Verification items for this drawing (mm, ordinates from the low corner). A direction names the side the tool comes from. Round coordinates to 2 decimals unless told otherwise and drop trailing zeros. Loops run counter-clockwise (first coordinate to the right, second up) from the corner with the lowest first, then second, coordinate; pieces in that order, holes last. Notation, with made-up numbers: (26, 3) - (63, 3) arc R21 cw to (63, 37) - close; hole circle Ø8 at (33, 73). An arc over 180 degrees is marked (long way). Put each result on its own line as item: value. Start each with the question number.
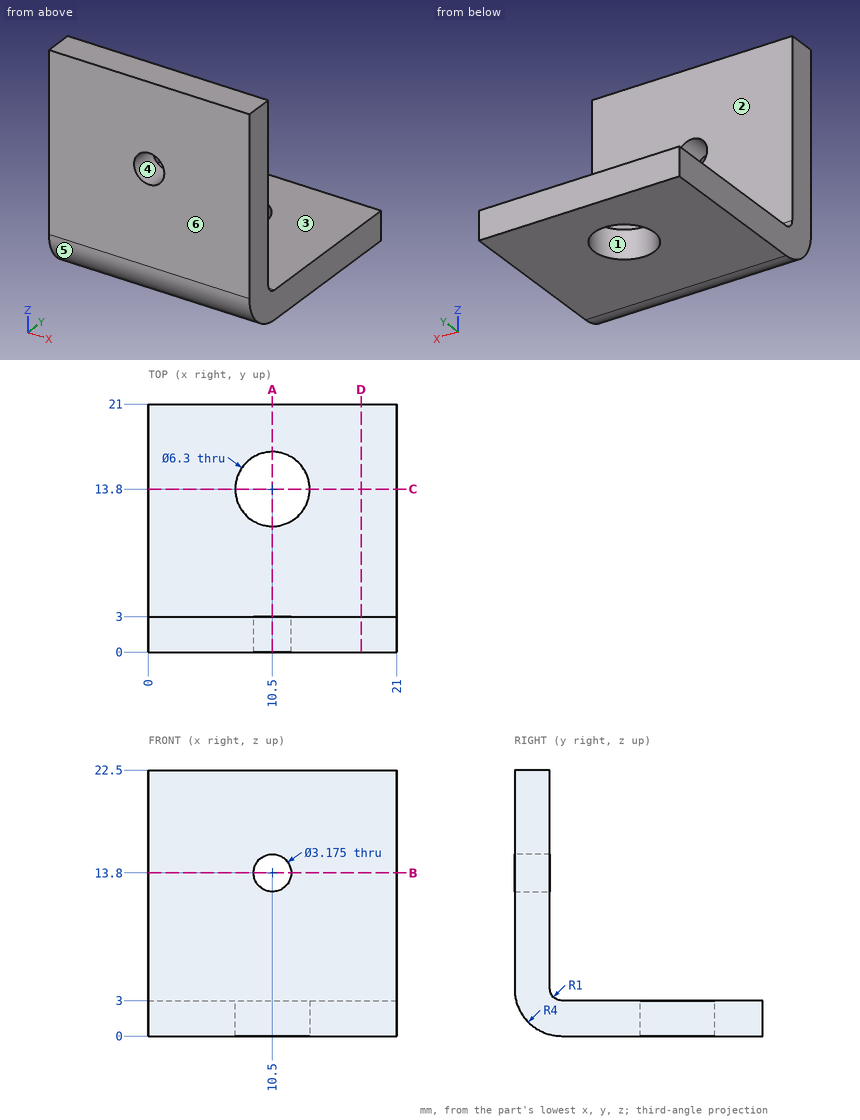
Q1. Depth check by flat-ended pin: pin 1 Ø8 at (y, z) = (14.5, 3.5) entering from +X. Enter the tip coordinate at first touch or a pass-through.
Q2. Cross-section at C-C on y = 13.8. Enter the section's corners in (x, z), and give its area (3 significant figures).
Q3. Draft check along Z on the marked faces 3, 4, 5 and 6. Enter one of: +Z half, -Z half, draft (parallel to the pull), parting line (faces both ways), or undercut.
Q4. Cross-section at A-A on x = 10.5. Enter the section's corners in (y, z), and give its area (3 significant figures).
Q5. Cross-section at D-D on x = 18. Enter the section's corners in (y, z), and give its area (3 significant figures).
Q6. Material ranges on line 1 (X direction, y = 2.1, z = 13.8); line 2 (Y direction, x = 14, z = 7), recorded low to high. Write a range as from..to.
Q7. Set-up check for the marked faces 1 and 2: record each of +Z, -Z, +X, -X, +Y, -Y from which the full face is reachable in a straight line by a thin tool's end or side.
Q8. Cross-section at B-B on z = 13.8. Enter the section's corners in (x, y), and give its area (3 significant figures).
Answer list:
1. pin 1: stops at x = 21
2. outline: (0, 0) - (7.35, 0) - (7.35, 3) - (0, 3) - close; (13.65, 0) - (21, 0) - (21, 3) - (13.65, 3) - close
2. area: 44.1 mm2
3. face 3: +Z half
3. face 4: undercut
3. face 5: -Z half
3. face 6: draft
4. outline: (0, 4) arc R4 ccw to (4, 0) - (10.65, 0) - (10.65, 3) - (4, 3) arc R1 cw to (3, 4) - (3, 12.21) - (0, 12.21) - close; (0, 15.39) - (3, 15.39) - (3, 22.5) - (0, 22.5) - close; (16.95, 0) - (21, 0) - (21, 3) - (16.95, 3) - close
4. area: 89.9 mm2
5. outline: (0, 4) arc R4 ccw to (4, 0) - (21, 0) - (21, 3) - (4, 3) arc R1 cw to (3, 4) - (3, 22.5) - (0, 22.5) - close
5. area: 118 mm2
6. line 1: x = 0..8.91, 12.09..21
6. line 2: y = 0..3
7. face 1: +Z, -Z
7. face 2: +Z, +X, -X, +Y
8. outline: (0, 0) - (8.91, 0) - (8.91, 3) - (0, 3) - close; (12.09, 0) - (21, 0) - (21, 3) - (12.09, 3) - close
8. area: 53.5 mm2
